```python
from build123d import *

# Parameters (mm, degrees)
F0_R           = 17
F0_R_2         = 7.5
F1_DEPTH       = 9
F3_SIZE        = 1
F2_R           = 2.5
F4_DEPTH       = 25
F5_R           = 6
F6_DEPTH       = 25
F6_DEPTH_BACK  = 25
F7_R           = 36.9830222821
F7_R_2         = 21.65
F8_DEPTH       = 25
F8_DEPTH_BACK  = 25
F9_R           = 5
F10_DEPTH      = 25
F10_DEPTH_BACK = 25
F12_DEPTH      = 25


with BuildPart() as f1:
    # F0 (on Right) → F1 (new body)
    with BuildSketch(Plane.YZ):
        Circle(F0_R)
        Circle(F0_R_2, mode=Mode.SUBTRACT)
    extrude(amount=F1_DEPTH)

    # F3
    f3_edges = [f1.edges().sort_by_distance(p)[0] for p in [
        (9, -17, 0),
    ]]
    chamfer(f3_edges, length=F3_SIZE)

    # F2 (on Top) → F4 (cut)
    with BuildSketch(Plane.XY):
        with Locations((4.5, 0)):
            Circle(F2_R)
    extrude(amount=F4_DEPTH, mode=Mode.SUBTRACT)

    # F5 (on Top) → F6 (join, two sides)
    with BuildSketch(Plane.XY) as f6_sk:
        with Locations((3.75, -14)):
            Circle(F5_R)
    extrude(amount=F6_DEPTH)
    extrude(f6_sk.sketch, amount=-F6_DEPTH_BACK)

    # F7 (on Right) → F8 (cut, two sides)
    with BuildSketch(Plane.YZ) as f8_sk:
        Circle(F7_R)
        Circle(F7_R_2, mode=Mode.SUBTRACT)
    extrude(amount=F8_DEPTH, mode=Mode.SUBTRACT)
    extrude(f8_sk.sketch, amount=-F8_DEPTH_BACK, mode=Mode.SUBTRACT)

    # F9 (on Top) → F10 (cut, two sides)
    with BuildSketch(Plane.XY) as f10_sk:
        with Locations((3.75, -14)):
            Circle(F9_R)
    extrude(amount=-F10_DEPTH, mode=Mode.SUBTRACT)
    extrude(f10_sk.sketch, amount=F10_DEPTH_BACK, mode=Mode.SUBTRACT)

    # F11 (on Right) → F12 (cut)
    with BuildSketch(Plane.YZ):
        with BuildLine():
            Line((-12, -6), (-12, 6))
            ThreePointArc((-12, 6), (-14, 8), (-16, 6))
            Line((-16, 6), (-16, -6))
            ThreePointArc((-16, -6), (-14, -8), (-12, -6))
        make_face()
    extrude(amount=-F12_DEPTH, mode=Mode.SUBTRACT)


solid = f1.part
```
CAD build for the part. Positions are in the model's coordinates, mm. A direction names the side the tool comes from. Round coordinates to 2 decimals unless told otherwise and drop trailing zeros. Order: outer loops, then holes, each group sorted by start corner. A loop starts at its lowest first (then second) coordinate and runs counter-clockwise, first axis right, second up.
Q1. Slice it at D-D (x = 6.5). Write the cut outline in (y, z).
Q2. Which spindle directions (+Z, -Z, +X, -X, +Y, -Y) get a long thin tool onto all of the face, cutting with end or side? Do faces 1 (the cylindrical face through (6.885, 0.751, 11.968)), 2 (the flat face through (9, 8, 0)), 3 (the cylindrical face through (4.44, -1.63, -7.32)), 4 (the cylindrical face through (-2, -14, 8)). Say none if no direction does.
Q3. Wall check: L1, parallel to Z at x = 7.25, y = 0; L2, parallel to X at y = -14, z = -8.25; L3, parallel to Y at x = 3.5, z = -4.5. Give the ranges that are in metal, low to high.
Q4. Two-plate mould, pull along Z, no slides. Class faces 5 (the conical face through (8.84, 16.15, -0.53)), 6 (the flat face through (0, 7, 4)), 7 (the cylindrical face through (-2, -14, -8)): pulls with the +Z half, pulls with the -Z half, needs draft (parallel to the pull), parting line crosses it, or undercut.
Q5. Slice it at B-B (x = 3.75). Write the cut outline in (y, z).
Q6. Slice it at A-A (y = -14). Write the cut outline in (x, z), and give its area (3 significant figures).
Q7. Slice it at C-C (y = 0). Write the cut outline in (x, z).
Q8. Drop flat-ended pins along their axis: pin 1 (4 mm diameter, centred on x = 4.5, y = 0, fed in from -Z); pin 2 (3 mm diameter, centred on x = 4.5, y = -12, fed in from +Z); pin 3 (6 mm diameter, centred on y = -4.5, z = -9.5, fed in from -X); pin 4 (2 mm diameter, centred on x = 4, z = -6.5, fed in from -Y). Give the stop position or say it passes through.
Results below:
1. outline: (-19.33, -9.75) arc R21.65 ccw to (-18.18, -11.76) - (-18.18, 11.76) arc R21.65 ccw to (-19.33, 9.75) - close; (-9.82, -19.29) arc R21.65 ccw to (-8.67, -19.84) - (-8.67, -14.62) arc R17 ccw (long way) to (1.5, 16.93) - (1.5, 7.35) arc R7.5 cw (long way) to (-1.5, 7.35) - (-1.5, 16.93) arc R17 ccw to (-8.67, 14.62) - (-8.67, 19.84) arc R21.65 ccw to (-9.82, 19.29) - close
2. face 1: +Z
2. face 2: +Z, -Z, +X, +Y
2. face 3: +X, -X
2. face 4: -X
3. L1: z = -17 to -7.5, 7.5 to 17
3. L2: x = -2.25 to -1.25, 8.75 to 9.75
3. L3: y = -19.99 to -18.99, -9.01 to -6, 6 to 16.39
4. face 5: parting line crosses it
4. face 6: needs draft
4. face 7: undercut
5. outline: (-20, -8.29) arc R21.65 ccw to (-19, -10.38) - (-19, 10.38) arc R21.65 ccw to (-20, 8.29) - close; (-9, -19.69) arc R21.65 ccw to (-8, -20.12) - (-8, -15) arc R17 ccw (long way) to (2.38, 16.83) - (2.38, 7.11) arc R7.5 cw (long way) to (-2.38, 7.11) - (-2.38, 16.83) arc R17 ccw to (-8, 15) - (-8, 20.12) arc R21.65 ccw to (-9, 19.69) - close
6. outline: (-2.25, -16.51) - (-1.25, -16.51) - (-1.25, -8) - (-2.25, -8) - close; (-2.25, 8) - (-1.25, 8) - (-1.25, 16.51) - (-2.25, 16.51) - close; (8.75, -16.51) - (9.75, -16.51) - (9.75, 16.51) - (8.75, 16.51) - close
6. area: 50.1 mm2
7. outline: (0, -17) - (8, -17) - (9, -16) - (9, -7.5) - (0, -7.5) - close; (0, 7.5) - (2, 7.5) - (2, 17) - (0, 17) - close; (7, 7.5) - (9, 7.5) - (9, 16) - (8, 17) - (7, 17) - close
8. pin 1: stops at z = -17
8. pin 2: passes through
8. pin 3: stops at x = 0
8. pin 4: stops at y = -20
